Check sheet for the modelled part. Datum: model origin and axes. Units: mm. A direction names the side the tool comes from. Give positions to 0.01 mm unless a question says otherwise; leave off trailing zeros. Order: outer loops, then holes, each group sorted by start corner. A loop starts at its lowest first (then second) coordinate and runs counter-clockwise, first axis right, second up.
```python
from build123d import *

# Parameters (mm, degrees)
F1_DEPTH = 157
F2_T     = -2
F3_R     = 11
F4_DEPTH = 157
F6_D     = 6
F7_R     = 7
F8_DEPTH = 3


with BuildPart() as f1:
    # F0 (on Front) → F1 (new body)
    with BuildSketch(Plane.XZ):
        Polygon((-20.5, 17), (-20.5, 0), (0, 0), (20.5, 0), (20.5, 17), (6.75, 32), (0, 32), (-6.75, 32), align=None)
    extrude(amount=-F1_DEPTH)

    # F2
    f2_openings = [f1.faces().sort_by_distance(p)[0] for p in [
        (0, 78.5, 0),
    ]]
    offset(amount=F2_T, openings=f2_openings)

    # F3 (on Front) → F4 (cut)
    with BuildSketch(Plane.XZ):
        with Locations((0, -9)):
            Circle(F3_R)
    extrude(amount=-F4_DEPTH, mode=Mode.SUBTRACT)

    # F6 (through all)
    with Locations(Plane(origin=(0, 0, 30), x_dir=(1, 0, 0), z_dir=(0, 0, -1))):
        with Locations((0, -18), (0, -77.5), (0, -137)):
            Hole(F6_D / 2)

    # F7 (on face) → F8 (cut)
    with BuildSketch(Plane(origin=(19.6075471698, 0, 17.9735849057), x_dir=(0, 1, 0), z_dir=(0.7371541402, 0, 0.6757246285))):
        with Locations((81.0107703245, 7.5740857882)):
            Circle(F7_R)
    extrude(amount=-F8_DEPTH, mode=Mode.SUBTRACT)


solid = f1.part
```
(1) Release check for a two-part mould opening along Y. For faces 3 (the face through (0, 157, 13)), 4 (the face through (-20.5, 77, 9)), 5 (the face through (-18.5, 77, 8)), 6 (the face through (-12.097, 77.429, 23.207)) record: released by +Y, released by -Y, zero draft, split by the parting line, or undercut.
Response values:
face 3: released by +Y
face 4: zero draft
face 5: undercut
face 6: undercut
(2) Cross-section at C-C on x = 0. Enter the section's corners in (y, z).
Response values:
outline: (0, 2) - (2, 2) - (2, 30) - (15, 30) - (15, 32) - (0, 32) - close; (21, 30) - (74.5, 30) - (74.5, 32) - (21, 32) - close; (80.5, 30) - (134, 30) - (134, 32) - (80.5, 32) - close; (140, 30) - (155, 30) - (155, 2) - (157, 2) - (157, 32) - (140, 32) - close
(3) Cross-section at A-A on z = 5. Enter the section's corners in (x, y), then the cut area to 3 significant figures.
Response values:
outline: (-20.5, 0) - (20.5, 0) - (20.5, 157) - (-20.5, 157) - close; hole (-18.5, 2) - (18.5, 2) - (18.5, 155) - (-18.5, 155) - close
area: 776 mm2
(4) Set-up check for faces 1 (the face through (-1.61, 134.47, 31.01)), 2 (the face through (8.06, 77.43, 27.61)): record each of +Z, -Z, +X, -X, +Y, -Y from which the full face is reachable in a straight line by a thin tool's end or side.
Response values:
face 1: +Z, -Z
face 2: -Z
(5) Cross-section at D-D on x = -9. Enter the section's corners in (y, z).
Response values:
outline: (0, 0) - (2, 0) - (2, 26.59) - (155, 26.59) - (155, 0) - (157, 0) - (157, 29.55) - (0, 29.55) - close
(6) Cross-section at B-B on y = 18. Enter the section's corners in (x, z).
Response values:
outline: (-20.5, 0) - (-18.5, 0) - (-18.5, 16.22) - (-5.87, 30) - (-3, 30) - (-3, 32) - (-6.75, 32) - (-20.5, 17) - close; (3, 30) - (5.87, 30) - (18.5, 16.22) - (18.5, 0) - (20.5, 0) - (20.5, 17) - (6.75, 32) - (3, 32) - close
(7) Material ranges on L1, parallel to Y at x = 0.5, z = 6.5; L2, parallel to X at y = 129, z = 11; L3, parallel to Z at x = 5, y = 22.5, recorded low to high.
Response values:
L1: y = 0 to 2, 155 to 157
L2: x = -20.5 to -18.5, 18.5 to 20.5
L3: z = 30 to 32
(8) Gauge pin test, flat ends, axial feed: pin 1 Ø5 at (x, y) = (13.5, 19.5) entering from +Z; pin 2 Ø15 at (x, z) = (3, 14) entering from -Y; pin 3 Ø9.5 at (x, y) = (0, 18) entering from -Z; pin 4 Ø9.5 at (x, y) = (2, 105) entering from -Z. Record the tip position at first contact, or that the pin passes through.
Response values:
pin 1: stops at z = 27.36
pin 2: stops at y = 0
pin 3: stops at z = 30
pin 4: stops at z = 29.04
